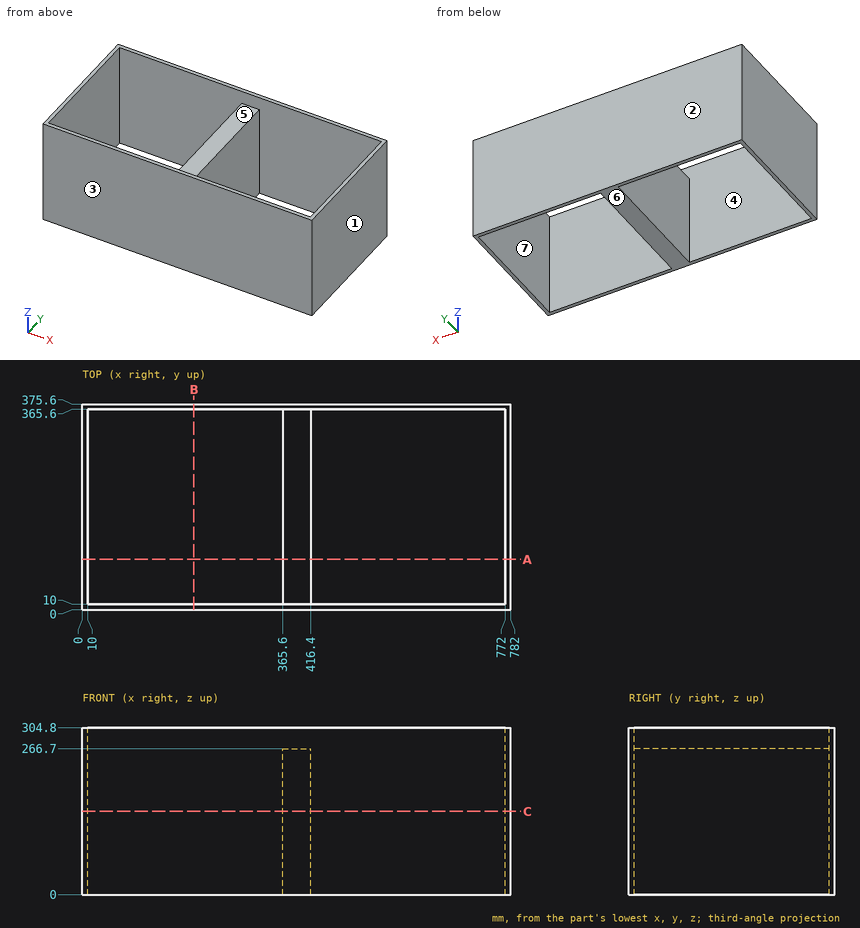
For this review, use the dimensioned drawing (mm, ordinates from the lowest corner) and the shaded views. A direction names the side the tool comes from. Give positions to 0.01 mm unless a question says otherwise; leave off trailing zeros. Loops run counter-clockwise (first coordinate to the right, second up) from the corner with the lowest first, then second, coordinate; pieces in that order, holes last.
Item 1: Tool access review of the marked faces 5, 6 and 7: name each direction out of +Z, -Z, +X, -X, +Y, -Y from which nothing blocks a thin tool from reaching the whole face with its end or side.
Item 2: For line 1 along X through (y, z) = (101, 262.5); line 2 along Y through (x, z) = (625.5, 116.5); line 3 along Z through (x, y) = (411, 209.5), list the stretches that pass through material, from the lowest coordinate up.
Item 3: Draft analysis for pull direction Y (two halves, no side actions). For the marked faces 1, 2, 3 and 4, state which applies: +Y half, -Y half, draft (parallel to the pull), parting line (faces both ways), or undercut.
Item 4: Take a section at C-C, the plane z = 152. State the section outline as (x, y) points.
Item 5: Take a section at B-B, the plane x = 203.5. State the section outline as (y, z) points.
Item 6: Take a section at A-A, the plane y = 92. State the section outline as (x, z) points, and give its area (3 significant figures).
Calculated:
1. face 5: +Z
1. face 6: -Z, +X, -X, +Y, -Y
1. face 7: +Z, -Z
2. line 1: x = 0 to 10, 365.6 to 416.4, 772 to 782
2. line 2: y = 0 to 10, 365.6 to 375.6
2. line 3: z = 0 to 266.7
3. face 1: draft
3. face 2: +Y half
3. face 3: -Y half
3. face 4: undercut
4. outline: (0, 0) - (782, 0) - (782, 375.6) - (0, 375.6) - close; hole (10, 10) - (365.6, 10) - (365.6, 365.6) - (10, 365.6) - close; hole (416.4, 10) - (772, 10) - (772, 365.6) - (416.4, 365.6) - close
5. outline: (0, 0) - (10, 0) - (10, 304.8) - (0, 304.8) - close; (365.6, 0) - (375.6, 0) - (375.6, 304.8) - (365.6, 304.8) - close
6. outline: (0, 0) - (10, 0) - (10, 304.8) - (0, 304.8) - close; (365.6, 0) - (416.4, 0) - (416.4, 266.7) - (365.6, 266.7) - close; (772, 0) - (782, 0) - (782, 304.8) - (772, 304.8) - close
6. area: 19,600 mm2
